Source: three-view drawing plus pictorial views. Frame: mm from the lowest corner of the part. A direction names the side the tool comes from. Round coordinates to 2 decimals unless told otherwise and drop trailing zeros. Loops run counter-clockwise (first coordinate to the right, second up) from the corner with the lowest first, then second, coordinate; pieces in that order, holes last. Notation, with made-up numbers: (18, 48.5) -> (77, 48.5) arc R12 cw to (77, 59.5) -> close; hole circle Ø9 at (-15, 33.5). An arc over 180 degrees is marked (long way). Put each result on its own line as item: value. Start each with the question number.
1. Cut plane D-D (z = 6.5). Return the cut outline in (x, y), then the cut area to 3 significant figures.
2. Cut plane A-A (y = 16.25). Return the cut outline in (x, z).
3. Set-up query: the marked faces 1, 2 and 3. Return all of +Z, -Z, +X, -X, +Y, -Y with unobstructed straight access to the full face (end or side cutting, diameter ignored); none if empty.
4. Cut plane B-B (z = 11.5). Return the cut outline in (x, y).
5. Contact query for flat-ended pins moving along their axis: pin 1 (4 mm diameter, centred on y = 16.5, z = 8, fed in from -X); pin 2 (4 mm diameter, centred on y = 17.5, z = 9.5, fed in from +X); pin 3 (5.5 mm diameter, centred on x = 23, y = 9.5, fed in from +Z). Output: stop coordinate, or through.
6. Cut plane C-C (x = 17). Return the cut outline in (y, z).
7. Material intervals for L1, parallel to X at y = 14.5, z = 4.25; L2, parallel to Y at x = 28, z = 10.75; L3, parallel to Z at x = 23.5, y = 18, sorted ascending.
8. Draft query along X for the marked faces 4, 5, 6 and 7. Return one class per face: pulls with the +X half, pulls with the -X half, needs draft (parallel to the pull), parting line crosses it, or undercut.
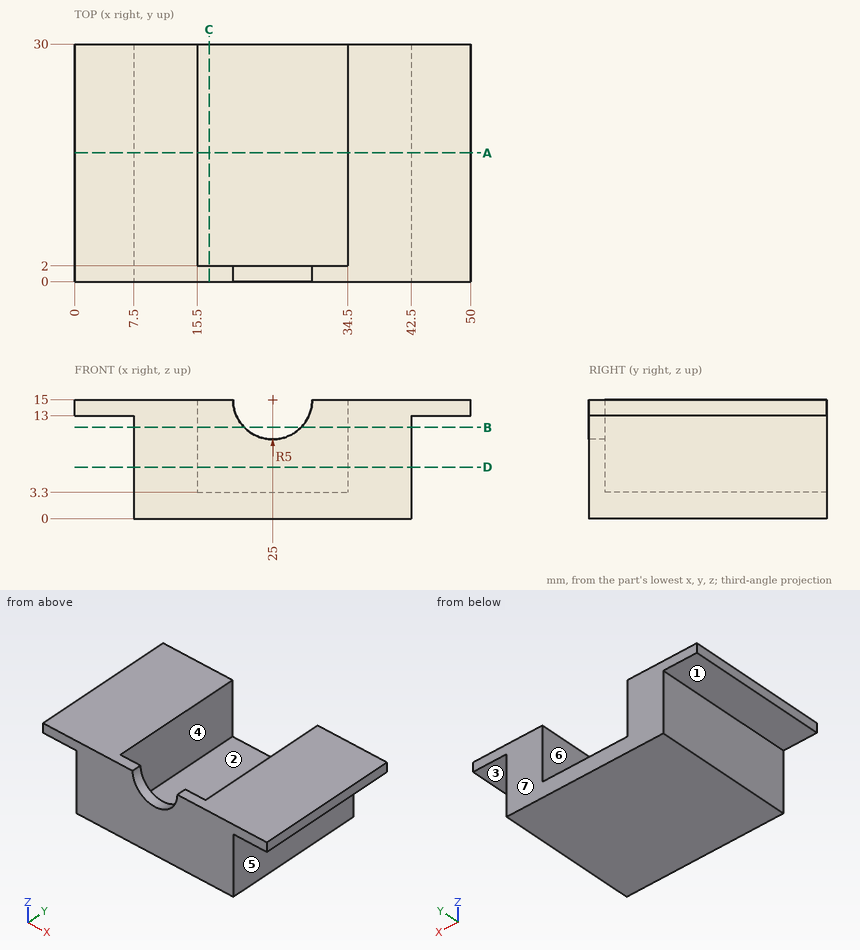
Solution:
1. outline: (7.5, 0) -> (42.5, 0) -> (42.5, 30) -> (34.5, 30) -> (34.5, 2) -> (15.5, 2) -> (15.5, 30) -> (7.5, 30) -> close
1. area: 518 mm^2
2. outline: (0, 13) -> (7.5, 13) -> (7.5, 0) -> (42.5, 0) -> (42.5, 13) -> (50, 13) -> (50, 15) -> (34.5, 15) -> (34.5, 3.3) -> (15.5, 3.3) -> (15.5, 15) -> (0, 15) -> close
3. face 1: -Z, -X, +Y, -Y
3. face 2: +Z, +Y
3. face 3: -Z, +X, +Y, -Y
4. outline: (7.5, 0) -> (21.43, 0) -> (21.43, 2) -> (15.5, 2) -> (15.5, 30) -> (7.5, 30) -> close; (28.57, 0) -> (42.5, 0) -> (42.5, 30) -> (34.5, 30) -> (34.5, 2) -> (28.57, 2) -> close
5. pin 1: stops at x = 7.5
5. pin 2: stops at x = 42.5
5. pin 3: stops at z = 3.3
6. outline: (0, 0) -> (30, 0) -> (30, 3.3) -> (2, 3.3) -> (2, 15) -> (0, 15) -> close
7. L1: x = 7.5 to 15.5, 34.5 to 42.5
7. L2: y = 0 to 2
7. L3: z = 0 to 3.3
8. face 4: undercut
8. face 5: pulls with the +X half
8. face 6: undercut
8. face 7: needs draft
